Check sheet for the modelled part. Datum: model origin and axes. Units: mm. A direction names the side the tool comes from. Give positions to 0.01 mm unless a question says otherwise; leave off trailing zeros. Write each loop counter-clockwise with the first axis right and the second up, starting at its lowest first coordinate (ties: lowest second). Pieces come first, ordered by that corner, then holes. Notation, with made-up numbers: M 6,-23.5 L 28,-23.5 A18 cw 28,-4.5 Z; hole C 19,74.25 d9. An arc over 180 degrees is marked long. Write item = value, one per line. Start each with the question number.
1) Cross-section at D-D, the plane y = -10.5. Record the cut outline in (x, z) (3 decimals), plus the area to 3 significant figures.
2) Mould release check, pull along Z, two halves, no side actions. Record for faces 1 (the flat face through (-37, -5.099, 6)), 2 (the flat face through (1.5, -7, 5)), 3 (the flat face through (-25, -7, 0)), 4 (the flat face through (-46, -5, 3)): released by +Z, released by -Z, zero draft, split by the parting line, or undercut.
3) Access from +Z, -Z, +X, -X, +Y, -Y to the whole of each face (thin tool, end or side, straight path). Record for faces 5 (the cylindrical face through (-48.997, -6.628, 6.549)), 6 (the flat face through (-25, -11.499, 5)), 7 (the flat face through (-9, -5.099, 6)).
4) Cross-section at C-C, the plane y = -7.25. Record the cut outline in (x, z) (3 decimals), plus the area to 3 significant figures.
5) Scan lines: line 1 along X through (y, z) = (-7, 7.5); line 2 along Y through (x, z) = (-3.25, 2.35); line 3 along X through (y, z) = (-9, 9). Record each from-to range of solid material in increasing order. Write a range as [from, to].
6) Cross-section at B-B, the plane z = 5.5. Record the cut outline in (x, y).
7) Cross-section at A-A, the plane x = -46.25. Record the cut outline in (y, z), plus the area to 4 significant figures.
8) Go/stop test with flat-tipped pins: pin 1 (3 mm diameter, centred on x = -2, y = -5.5, fed in from +Z); pin 2 (1.6 mm diameter, centred on x = -38.75, z = 5, fed in from -Y); pin 3 (3 mm diameter, centred on x = -46.25, y = -6.75, fed in from +Z); pin 4 (3 mm diameter, centred on x = -39.5, z = 4.5, fed in from +Y). Record where each tip stops, or that it passes through.
```python
from build123d import *

# Parameters (mm, degrees)
SKETCH1_W           = 52.5
SKETCH1_H           = 9.5
SKETCH1_R           = 1.375
BOSS_EXTRUDE1_DEPTH = 10
SKETCH4_R           = 2.75
CUT_EXTRUDE3_DEPTH  = 7
CUT_EXTRUDE1_REACH  = 54.832
SKETCH2_R           = 1.375
SKETCH3_R           = 2.75
CUT_EXTRUDE2_DEPTH  = 3.1


with BuildPart() as part:
    # Sketch1 → Boss-Extrude1 (new body)
    with BuildSketch(Plane.XY):
        with Locations((-24.75, -6.748746096)):
            Rectangle(SKETCH1_W, SKETCH1_H)
        with Locations((-46.25, -6.748746096)):
            Circle(SKETCH1_R, mode=Mode.SUBTRACT)
        with Locations((-3.25, -6.748746096)):
            Circle(SKETCH1_R, mode=Mode.SUBTRACT)
    extrude(amount=BOSS_EXTRUDE1_DEPTH)

    # Sketch4 → Cut-Extrude3 (cut)
    with BuildSketch(Plane.XY.offset(10)):
        with Locations((-46.25, -6.748746096)):
            Circle(SKETCH4_R)
        with Locations((-3.25, -6.748746096)):
            Circle(SKETCH4_R)
    extrude(amount=-CUT_EXTRUDE3_DEPTH, mode=Mode.SUBTRACT)

    # Sketch2 → Cut-Extrude1 (cut, up to next)
    with BuildSketch(Plane(origin=(0, -1.998746096, 0), x_dir=(1, 0, 0), z_dir=(0, 1, 0)), mode=Mode.PRIVATE) as cut_extrude1_sk1:
        with Locations(Location((-10.75, -5, 0), (0, 0, 270))):
            Circle(SKETCH2_R)
    cut_extrude1_tool1 = extrude(cut_extrude1_sk1.sketch, amount=-CUT_EXTRUDE1_REACH, mode=Mode.PRIVATE) & part.part
    # Sketch2 → Cut-Extrude1 (cut, up to next)
    with BuildSketch(Plane(origin=(0, -1.998746096, 0), x_dir=(1, 0, 0), z_dir=(0, 1, 0)), mode=Mode.PRIVATE) as cut_extrude1_sk2:
        with Locations(Location((-38.75, -5, 0), (0, 0, 270))):
            Circle(SKETCH2_R)
    cut_extrude1_tool2 = extrude(cut_extrude1_sk2.sketch, amount=-CUT_EXTRUDE1_REACH, mode=Mode.PRIVATE) & part.part
    add(cut_extrude1_tool1.solids().sort_by_distance((-10.75, -1.998746, 5))[0], mode=Mode.SUBTRACT)
    add(cut_extrude1_tool2.solids().sort_by_distance((-38.75, -1.998746, 5))[0], mode=Mode.SUBTRACT)

    # Sketch3 → Cut-Extrude2 (cut)
    with BuildSketch(Plane(origin=(0, -1.998746096, 0), x_dir=(1, 0, 0), z_dir=(0, 1, 0))):
        with Locations(Location((-10.75, -5, 0), (0, 0, 270))):
            Circle(SKETCH3_R)
        with Locations(Location((-38.75, -5, 0), (0, 0, 270))):
            Circle(SKETCH3_R)
    extrude(amount=-CUT_EXTRUDE2_DEPTH, mode=Mode.SUBTRACT)


solid = part.part
```
Reply:
q1.outline = M -51,0 L 1.5,0 L 1.5,10 L -51,10 Z; hole C -38.75,5 d2.75; hole C -10.75,5 d2.75
q1.area = 513 mm2
q2.face_1 = undercut
q2.face_2 = zero draft
q2.face_3 = released by -Z
q2.face_4 = released by +Z
q3.face_5 = +Z
q3.face_6 = +Z, -Z, +X, -X, -Y
q3.face_7 = +Y
q4.outline = M -51,0 L -47.53,0 L -47.53,3 L -48.954,3 L -48.954,10 L -51,10 Z; M -44.97,0 L -4.53,0 L -4.53,3 L -5.954,3 L -5.954,10 L -43.546,10 L -43.546,3 L -44.97,3 Z; M -1.97,0 L 1.5,0 L 1.5,10 L -0.546,10 L -0.546,3 L -1.97,3 Z; hole C -38.75,5 d2.75; hole C -10.75,5 d2.75
q4.area = 422 mm2
q5.line_1 = [-51, -48.99], [-43.51, -5.99], [-0.51, 1.5]
q5.line_2 = [-11.5, -8.12], [-5.37, -2]
q5.line_3 = [-51, -47.83], [-44.67, -4.83], [-1.67, 1.5]
q6.outline = M -51,-11.5 L -40.03,-11.5 L -40.03,-5.1 L -41.45,-5.1 L -41.45,-2 L -51,-2 Z; M -37.47,-11.5 L -12.03,-11.5 L -12.03,-5.1 L -13.45,-5.1 L -13.45,-2 L -36.05,-2 L -36.05,-5.1 L -37.47,-5.1 Z; M -9.47,-11.5 L 1.5,-11.5 L 1.5,-2 L -8.05,-2 L -8.05,-5.1 L -9.47,-5.1 Z; hole C -46.25,-6.75 d5.5; hole C -3.25,-6.75 d5.5
q7.outline = M -11.5,0 L -8.12,0 L -8.12,3 L -9.5,3 L -9.5,10 L -11.5,10 Z; M -5.37,0 L -2,0 L -2,10 L -4,10 L -4,3 L -5.37,3 Z
q7.area = 48.25 mm2
q8.pin_1 = 10
q8.pin_2 = through
q8.pin_3 = 3
q8.pin_4 = -5.1
